from build123d import *

# Parameters (mm, degrees)
SKETCH_1_R          = 2.5
SKETCH_1_R_2        = 1
EXTRUDE_1_DEPTH     = 3
SKETCH_2_R          = 3.4
SKETCH_2_R_2        = 2.5
EXTRUDE_2_DEPTH     = 2.2
CUT_EXTRUDE_1_DEPTH = 2
SKETCH_5_R          = 3
CUT_EXTRUDE_2_DEPTH = 1


with BuildPart() as part:
    # 草图1 → 凸台-拉伸1 (new body)
    with BuildSketch(Plane.XY):
        with BuildLine():
            Line((-6.505574533, 2.8), (-4.38178046, 2.8))
            ThreePointArc((-4.38178046, 2.8), (-3.966553061, 2.890282348), (-3.62630107, 3.144827586))
            ThreePointArc((-3.62630107, 3.144827586), (0, 4.8), (3.62630107, 3.144827586))
            ThreePointArc((3.62630107, 3.144827586), (3.966553061, 2.890282348), (4.38178046, 2.8))
            Line((4.38178046, 2.8), (6.505574533, 2.8))
            ThreePointArc((6.505574533, 2.8), (7.111104603, 2.595822426), (7.469363352, 2.066666667))
            ThreePointArc((7.469363352, 2.066666667), (7.75, 0), (7.469363352, -2.066666667))
            ThreePointArc((7.469363352, -2.066666667), (7.111104603, -2.595822426), (6.505574533, -2.8))
            Line((6.505574533, -2.8), (4.38178046, -2.8))
            ThreePointArc((4.38178046, -2.8), (3.966553061, -2.890282348), (3.62630107, -3.144827586))
            ThreePointArc((3.62630107, -3.144827586), (0, -4.8), (-3.62630107, -3.144827586))
            ThreePointArc((-3.62630107, -3.144827586), (-3.966553061, -2.890282348), (-4.38178046, -2.8))
            Line((-4.38178046, -2.8), (-6.505574533, -2.8))
            ThreePointArc((-6.505574533, -2.8), (-7.111104603, -2.595822426), (-7.469363352, -2.066666667))
            ThreePointArc((-7.469363352, -2.066666667), (-7.75, 0), (-7.469363352, 2.066666667))
            ThreePointArc((-7.469363352, 2.066666667), (-7.111104603, 2.595822426), (-6.505574533, 2.8))
        make_face()
        Circle(SKETCH_1_R, mode=Mode.SUBTRACT)
        with Locations((-5.5, 0)):
            Circle(SKETCH_1_R_2, mode=Mode.SUBTRACT)
        with Locations(Location((5.5, 0, 0), (0, 0, 180))):
            Circle(SKETCH_1_R_2, mode=Mode.SUBTRACT)
    extrude(amount=EXTRUDE_1_DEPTH)

    # 草图2 → 凸台-拉伸2 (add)
    with BuildSketch(Plane.XY.offset(3)):
        Circle(SKETCH_2_R)
        Circle(SKETCH_2_R_2, mode=Mode.SUBTRACT)
    extrude(amount=EXTRUDE_2_DEPTH)

    # 草图4 → 切除-拉伸1 (cut)
    with BuildSketch(Plane(origin=(0, 0, 0), x_dir=(-1, 0, 0), z_dir=(0, 0, -1))):
        with BuildLine():
            Line((-5.5, 2), (-7.487489566, 2))
            ThreePointArc((-7.487489566, 2), (-7.75, 0), (-7.487489566, -2))
            Line((-7.487489566, -2), (-5.5, -2))
            ThreePointArc((-5.5, -2), (-3.5, 0), (-5.5, 2))
        make_face()
        with BuildLine():
            Line((5.5, -2), (7.487489566, -2))
            ThreePointArc((7.487489566, -2), (7.75, 0), (7.487489566, 2))
            Line((7.487489566, 2), (5.5, 2))
            ThreePointArc((5.5, 2), (3.5, 0), (5.5, -2))
        make_face()
    extrude(amount=-CUT_EXTRUDE_1_DEPTH, mode=Mode.SUBTRACT)

    # 草图5 → 切除-拉伸2 (cut)
    with BuildSketch(Plane.XY.offset(5.2)):
        Circle(SKETCH_5_R)
    extrude(amount=-CUT_EXTRUDE_2_DEPTH, mode=Mode.SUBTRACT)


solid = part.part
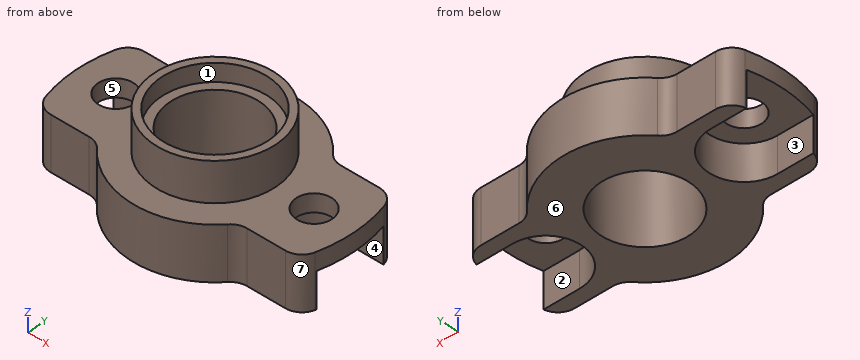
Could you check a few things on this model? Use its own coordinates, in mm. Face numbers are marked on the shaded views. A direction names the side the tool comes from. Give positions to 0.01 mm unless a question says otherwise; leave off trailing zeros. Loops run counter-clockwise (first coordinate to the right, second up) from the corner with the lowest first, then second, coordinate; pieces in that order, holes last. Notation, with made-up numbers: (36, -31.5) -> (78, -31.5) arc R19 ccw to (78, -21.5) -> close; hole circle Ø2 at (89, 70.25). An arc over 180 degrees is marked (long way). Return JSON: item names as keys, results as strings.
Item 1: If we section it at D-D on z = 1.35: List the corners of the cut face in (x, y) for me.
Geometry results:
{"outline": "(-7.49, -2) arc R7.75 ccw to (-7.47, -2.07) arc R1 ccw to (-6.51, -2.8) -> (-4.38, -2.8) arc R1 cw to (-3.63, -3.14) arc R4.8 ccw to (3.63, -3.14) arc R1 cw to (4.38, -2.8) -> (6.51, -2.8) arc R1 ccw to (7.47, -2.07) arc R7.75 ccw to (7.49, -2) -> (5.5, -2) arc R2 cw to (5.5, 2) -> (7.49, 2) arc R7.75 ccw to (7.47, 2.07) arc R1 ccw to (6.51, 2.8) -> (4.38, 2.8) arc R1 cw to (3.63, 3.14) arc R4.8 ccw to (-3.63, 3.14) arc R1 cw to (-4.38, 2.8) -> (-6.51, 2.8) arc R1 ccw to (-7.47, 2.07) arc R7.75 ccw to (-7.49, 2) -> (-5.5, 2) arc R2 cw to (-5.5, -2) -> close; hole circle Ø5 at (0, 0)"}
Item 2: I need wall thicknesses on L1, parallel to Y at x = 0, z = 4.85; L2, parallel to Y at x = -5.5, z = 2.6; L3, parallel to X at y = 0, z = 1.85. Which ranges of each line are inside material? Lowest first, please. Write a range as from..to.
Geometry results:
{"L1": "y = -3.4..-3, 3..3.4", "L2": "y = -2.8..-1, 1..2.8", "L3": "x = -3.5..-2.5, 2.5..3.5"}
Item 3: If we section it at C-C on y = 0: List the corners of the cut face in (x, z) for me, plus the area to 3 significant figures.
Geometry results:
{"outline": "(-7.75, 2) -> (-6.5, 2) -> (-6.5, 3) -> (-7.75, 3) -> close; (-4.5, 2) -> (-3.5, 2) -> (-3.5, 0) -> (-2.5, 0) -> (-2.5, 4.2) -> (-3, 4.2) -> (-3, 5.2) -> (-3.4, 5.2) -> (-3.4, 3) -> (-4.5, 3) -> close; (2.5, 0) -> (3.5, 0) -> (3.5, 2) -> (4.5, 2) -> (4.5, 3) -> (3.4, 3) -> (3.4, 5.2) -> (3, 5.2) -> (3, 4.2) -> (2.5, 4.2) -> close; (6.5, 2) -> (7.75, 2) -> (7.75, 3) -> (6.5, 3) -> close", "area": "13.5 mm²"}
Item 4: If we section it at A-A on x = 0: List the corners of the cut face in (y, z) for me.
Geometry results:
{"outline": "(-4.8, 0) -> (-2.5, 0) -> (-2.5, 4.2) -> (-3, 4.2) -> (-3, 5.2) -> (-3.4, 5.2) -> (-3.4, 3) -> (-4.8, 3) -> close; (2.5, 0) -> (4.8, 0) -> (4.8, 3) -> (3.4, 3) -> (3.4, 5.2) -> (3, 5.2) -> (3, 4.2) -> (2.5, 4.2) -> close"}
Item 5: Which directions (+Z, -Z, +X, -X, +Y, -Y) give clear straight access to the entire face, cutting with the end or side of a thin tool? Please do the marked faces 1, 2 and 3.
Geometry results:
{"face 1": "+Z", "face 2": "-Z, +X", "face 3": "-Z, -X"}
Item 6: We'd pull the mould along Y, two halves only. Please class the marked faces 4, 5, 6 and 7: +Y half, -Y half, draft (parallel to the pull), parting line (faces both ways), or undercut.
Geometry results:
{"face 4": "undercut", "face 5": "undercut", "face 6": "draft", "face 7": "-Y half"}
Item 7: If we section it at B-B on z = 2.7: List the corners of the cut face in (x, y) for me, plus the area to 3 significant figures.
Geometry results:
{"outline": "(-7.47, -2.07) arc R1 ccw to (-6.51, -2.8) -> (-4.38, -2.8) arc R1 cw to (-3.63, -3.14) arc R4.8 ccw to (3.63, -3.14) arc R1 cw to (4.38, -2.8) -> (6.51, -2.8) arc R1 ccw to (7.47, -2.07) arc R7.75 ccw to (7.47, 2.07) arc R1 ccw to (6.51, 2.8) -> (4.38, 2.8) arc R1 cw to (3.63, 3.14) arc R4.8 ccw to (-3.63, 3.14) arc R1 cw to (-4.38, 2.8) -> (-6.51, 2.8) arc R1 ccw to (-7.47, 2.07) arc R7.75 ccw to start; hole circle Ø2 at (-5.5, 0); hole circle Ø5 at (0, 0); hole circle Ø2 at (5.5, 0)", "area": "80.5 mm²"}
Item 8: I'm going to push flat-ended pins straight in: pin 1 (2 mm diameter, centred on x = 6, y = 0.5, fed in from -Z); pin 2 (3 mm diameter, centred on x = -5.5, y = 0, fed in from +Z); pin 3 (0.6 mm diameter, centred on x = 5.5, z = 1, fed in from -Y). Where does each tip first touch, or does it pass through?
Geometry results:
{"pin 1": "stops at z = 2", "pin 2": "stops at z = 3", "pin 3": "stops at y = -2.8"}
